```python
from build123d import *

# Parameters (mm, degrees)
SKETCH_1_R      = 1.5
EXTRUDE_1_DEPTH = 2.5


with BuildPart() as part:
    # 草图1 → 凸台-拉伸1 (new body)
    with BuildSketch(Plane(origin=(0, 0, 0), x_dir=(1, 0, 0), z_dir=(0, 1, 0))):
        with BuildLine():
            Line((3.882285677, 14.488887394), (3.364647586, 12.557035742))
            ThreePointArc((3.364647586, 12.557035742), (5.405611466, 13.028620317), (7.5, 12.990381057))
            Line((7.5, 12.990381057), (6.5, 11.258330249))
            ThreePointArc((6.5, 11.258330249), (8.593474792, 11.185605648), (10.606601718, 10.606601718))
            Line((10.606601718, 10.606601718), (9.192388155, 9.192388155))
            ThreePointArc((9.192388155, 9.192388155), (11.195707011, 8.580310438), (12.990381057, 7.5))
            Line((12.990381057, 7.5), (11.258330249, 6.5))
            ThreePointArc((11.258330249, 6.5), (13.0349703, 5.390281252), (14.488887394, 3.882285677))
            Line((14.488887394, 3.882285677), (12.557035742, 3.364647586))
            ThreePointArc((12.557035742, 3.364647586), (13.985921904, 1.832913306), (15, 0))
            Line((15, 0), (13, 0))
            ThreePointArc((13, 0), (13.983756043, -1.849364653), (14.488887394, -3.882285677))
            Line((14.488887394, -3.882285677), (12.557035742, -3.364647586))
            ThreePointArc((12.557035742, -3.364647586), (13.028620317, -5.405611466), (12.990381057, -7.5))
            Line((12.990381057, -7.5), (11.258330249, -6.5))
            ThreePointArc((11.258330249, -6.5), (11.185605648, -8.593474792), (10.606601718, -10.606601718))
            Line((10.606601718, -10.606601718), (9.192388155, -9.192388155))
            ThreePointArc((9.192388155, -9.192388155), (8.580310438, -11.195707011), (7.5, -12.990381057))
            Line((7.5, -12.990381057), (6.5, -11.258330249))
            ThreePointArc((6.5, -11.258330249), (5.390281252, -13.0349703), (3.882285677, -14.488887394))
            Line((3.882285677, -14.488887394), (3.364647586, -12.557035742))
            ThreePointArc((3.364647586, -12.557035742), (1.832913306, -13.985921904), (0, -15))
            Line((0, -15), (0, -13))
            ThreePointArc((0, -13), (-1.849364653, -13.983756043), (-3.882285677, -14.488887394))
            Line((-3.882285677, -14.488887394), (-3.364647586, -12.557035742))
            ThreePointArc((-3.364647586, -12.557035742), (-5.405611466, -13.028620317), (-7.5, -12.990381057))
            Line((-7.5, -12.990381057), (-6.5, -11.258330249))
            ThreePointArc((-6.5, -11.258330249), (-8.593474792, -11.185605648), (-10.606601718, -10.606601718))
            Line((-10.606601718, -10.606601718), (-9.192388155, -9.192388155))
            ThreePointArc((-9.192388155, -9.192388155), (-11.195707011, -8.580310438), (-12.990381057, -7.5))
            Line((-12.990381057, -7.5), (-11.258330249, -6.5))
            ThreePointArc((-11.258330249, -6.5), (-13.0349703, -5.390281252), (-14.488887394, -3.882285677))
            Line((-14.488887394, -3.882285677), (-12.557035742, -3.364647586))
            ThreePointArc((-12.557035742, -3.364647586), (-13.985921904, -1.832913306), (-15, 0))
            Line((-15, 0), (-13, 0))
            ThreePointArc((-13, 0), (-13.983756043, 1.849364653), (-14.488887394, 3.882285677))
            Line((-14.488887394, 3.882285677), (-12.557035742, 3.364647586))
            ThreePointArc((-12.557035742, 3.364647586), (-13.028620317, 5.405611466), (-12.990381057, 7.5))
            Line((-12.990381057, 7.5), (-11.258330249, 6.5))
            ThreePointArc((-11.258330249, 6.5), (-11.185605648, 8.593474792), (-10.606601718, 10.606601718))
            Line((-10.606601718, 10.606601718), (-9.192388155, 9.192388155))
            ThreePointArc((-9.192388155, 9.192388155), (-8.580310438, 11.195707011), (-7.5, 12.990381057))
            Line((-7.5, 12.990381057), (-6.5, 11.258330249))
            ThreePointArc((-6.5, 11.258330249), (-5.390281252, 13.0349703), (-3.882285677, 14.488887394))
            Line((-3.882285677, 14.488887394), (-3.364647586, 12.557035742))
            ThreePointArc((-3.364647586, 12.557035742), (-1.832913306, 13.985921904), (0, 15))
            Line((0, 15), (0, 13))
            ThreePointArc((0, 13), (1.849364653, 13.983756043), (3.882285677, 14.488887394))
        make_face()
        with Locations((-10, 0)):
            Circle(SKETCH_1_R, mode=Mode.SUBTRACT)
        Circle(SKETCH_1_R, mode=Mode.SUBTRACT)
    extrude(amount=EXTRUDE_1_DEPTH)


solid = part.part
```
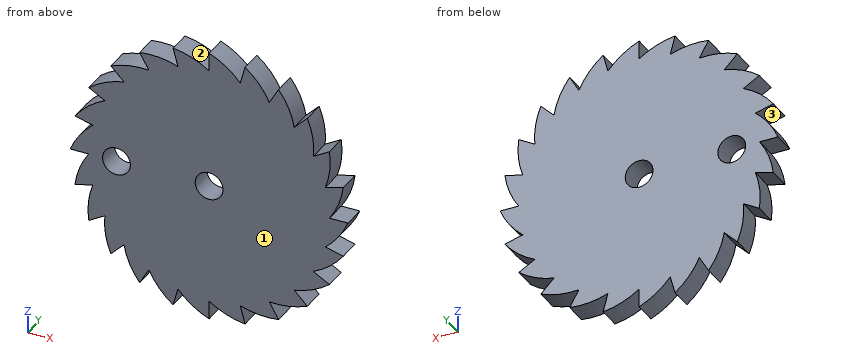
The model under review builds one solid part; all positions refer to its coordinate system, in mm. Face numbers are marked on the shaded views. Coordinates: 2 decimals unless noted, no trailing zeros. Write each loop counter-clockwise with the first axis right and the second up, starting at its lowest first coordinate (ties: lowest second). Pieces come first, ordered by that corner, then holes.
1) To check wall thickness, follow probe 1 along Z at (x, y) = (-13.25, 0.3); probe 2 along Z at (x, y) = (-7.25, 1.6); probe 3 along Z at (x, y) = (-10, 0.7). State the ranges of each line that lie inside material, in increasing order.
2) We need section D-D on y = 1.4. Count the separate pieces of the cut face and the enclosed holes in it, then the cut area to 3 significant figures.
3) We need section B-B on x = 1. State the section outline as (y, z) points, then the cut area to 3 significant figures.
4) We need section C-C on z = 10. State the section outline as (x, y) points.
5) We need section A-A on x = -10. State the section outline as (y, z) points.
6) Clearance check with flat-ended pins moving along their axes: pin 1 Ø0.6 at (y, z) = (1.5, -13.5) entering from +X; pin 2 Ø1.8 at (x, z) = (-10, 0) entering from -Y; pin 3 Ø1.5 at (x, y) = (2.5, 0.5) entering from -Z; pin 4 Ø1.5 at (y, z) = (1, -6) entering from -X. State where each tip first meets the part, or that it passes through.
7) The part is to be moulded in two halves that separate along X. For the marked faces 1, 2 and 3, say which applies: pulls with the +X half, pulls with the -X half, needs draft (parallel to the pull), parting line crosses it, or undercut.
Answer list:
1. probe 1: z = -3.55 to -0.38, 0 to 2.72, 3.55 to 5.21
1. probe 2: z = -12.56 to 11.29, 12.56 to 13.02
1. probe 3: z = -10 to -1.5, 1.5 to 9.01, 10 to 10.84
2. separate pieces: 1
2. enclosed holes: 2
2. area: 609 mm2
3. outline: (0, -13.6) - (2.5, -13.6) - (2.5, -1.12) - (0, -1.12) - close; (0, 1.12) - (2.5, 1.12) - (2.5, 14.52) - (0, 14.52) - close
3. area: 64.7 mm2
4. outline: (-10, 0) - (9.01, 0) - (9.01, 2.5) - (-10, 2.5) - close; (10, 0) - (10.84, 0) - (10.84, 2.5) - (10, 2.5) - close
5. outline: (0, -10) - (2.5, -10) - (2.5, -1.5) - (0, -1.5) - close; (0, 1.5) - (2.5, 1.5) - (2.5, 9.01) - (0, 9.01) - close; (0, 10) - (2.5, 10) - (2.5, 10.84) - (0, 10.84) - close
6. pin 1: stops at x = 3.7
6. pin 2: passes through
6. pin 3: stops at z = -14.39
6. pin 4: stops at x = -13.08
7. face 1: needs draft
7. face 2: undercut
7. face 3: pulls with the -X half
